Input: part model. Units: mm. Frame: model coordinates. Round coordinates to 2 decimals unless told otherwise and drop trailing zeros. Loops run counter-clockwise (first coordinate to the right, second up) from the corner with the lowest first, then second, coordinate; pieces in that order, holes last.
1) Section B-B, the plane y = 0.2. State how many separate pieces and enclosed holes the cut face has, and give its area (3 significant figures).
2) Section A-A, the plane x = 11.5. Return loops of the section in (y, z) (3 decimals), and give its area (3 significant figures).
3) First-contact query: pin 1 (0.6 mm diameter, centred on x = -26.5, y = 1, fed in from +Z); pin 2 (0.6 mm diameter, centred on x = -28, y = 0.5, fed in from -Z). Flat tips, straight axial feed; report the tip coordinate or a pass-through.
4) Ray query, line 1 along Z through (x, y) = (-25, 0.1); line 2 along X through (y, z) = (0, 7); line 3 along Z through (x, y) = (2.5, 1). Return the intervals inside material, ascending.
from build123d import *

# Parameters (mm, degrees)
SKETCH1_R           = 7.6
BOSS_EXTRUDE1_DEPTH = 1.8
FILLET1_R           = 3
FILLET2_R           = 1.4
SCALE1_SCALE        = 1.15


with BuildPart() as part:
    # Sketch1 → Boss-Extrude1 (new body)
    with BuildSketch(Plane(origin=(0, 0, 0), x_dir=(1, 0, 0), z_dir=(0, 1, 0))):
        Polygon((20.3, 35.160631394), (-20.3, 35.160631394), (-40.6, 0), (-20.3, -35.160631394), (20.3, -35.160631394), (40.6, 0), align=None)
        Polygon((-16.584596387, -31.040676977), (-16.771232891, -33.649562724), (-19.310104532, -34.278250893), (-20.692576995, -32.057915803), (-19.008120326, -30.056985082), align=None, mode=Mode.SUBTRACT)
        Polygon((-35.174313007, -1.157656706), (-37.526992591, -2.300467626), (-39.340888337, -0.416084372), (-38.109257976, 1.891339446), (-35.534172805, 1.433022539), align=None, mode=Mode.SUBTRACT)
        Polygon((18.589716619, -29.883020272), (20.7557597, -31.349095098), (20.030783805, -33.862166521), (17.41668098, -33.94925525), (16.52605248, -31.490007621), align=None, mode=Mode.SUBTRACT)
        with BuildLine():
            Line((-32.142053523, 3.218057696), (-18.857946477, 26.226806032))
            Line((-18.857946477, 26.226806032), (-10.521325069, 11.78735419))
            ThreePointArc((-10.521325069, 11.78735419), (-13.68320138, 7.9), (-15.468810706, 3.218057696))
            Line((-15.468810706, 3.218057696), (-32.142053523, 3.218057696))
        make_face(mode=Mode.SUBTRACT)
        with BuildLine():
            Line((-18.857946477, -26.226806032), (-32.142053523, -3.218057696))
            Line((-32.142053523, -3.218057696), (-15.468810706, -3.218057696))
            ThreePointArc((-15.468810706, -3.218057696), (-13.68320138, -7.9), (-10.521325069, -11.78735419))
            Line((-10.521325069, -11.78735419), (-18.857946477, -26.226806032))
        make_face(mode=Mode.SUBTRACT)
        with BuildLine():
            Line((13.284107046, -29.444863729), (-13.284107046, -29.444863729))
            Line((-13.284107046, -29.444863729), (-4.947485637, -15.005411886))
            ThreePointArc((-4.947485637, -15.005411886), (0, -15.8), (4.947485637, -15.005411886))
            Line((4.947485637, -15.005411886), (13.284107046, -29.444863729))
        make_face(mode=Mode.SUBTRACT)
        with BuildLine():
            Line((32.142053523, -3.218057696), (18.857946477, -26.226806032))
            Line((18.857946477, -26.226806032), (10.521325069, -11.78735419))
            ThreePointArc((10.521325069, -11.78735419), (13.68320138, -7.9), (15.468810706, -3.218057696))
            Line((15.468810706, -3.218057696), (32.142053523, -3.218057696))
        make_face(mode=Mode.SUBTRACT)
        with BuildLine():
            Line((18.857946477, 26.226806032), (32.142053523, 3.218057696))
            Line((32.142053523, 3.218057696), (15.468810706, 3.218057696))
            ThreePointArc((15.468810706, 3.218057696), (13.68320138, 7.9), (10.521325069, 11.78735419))
            Line((10.521325069, 11.78735419), (18.857946477, 26.226806032))
        make_face(mode=Mode.SUBTRACT)
        with BuildLine():
            Line((-13.284107046, 29.444863729), (13.284107046, 29.444863729))
            Line((13.284107046, 29.444863729), (4.947485637, 15.005411886))
            ThreePointArc((4.947485637, 15.005411886), (0, 15.8), (-4.947485637, 15.005411886))
            Line((-4.947485637, 15.005411886), (-13.284107046, 29.444863729))
        make_face(mode=Mode.SUBTRACT)
        Polygon((-18.589716619, 29.883020272), (-20.7557597, 31.349095098), (-20.030783805, 33.862166521), (-17.41668098, 33.94925525), (-16.52605248, 31.490007621), align=None, mode=Mode.SUBTRACT)
        Polygon((35.174313007, 1.157656706), (37.526992591, 2.300467626), (39.340888337, 0.416084372), (38.109257976, -1.891339446), (35.534172805, -1.433022539), align=None, mode=Mode.SUBTRACT)
        Polygon((16.584596387, 31.040676977), (16.771232891, 33.649562724), (19.310104532, 34.278250893), (20.692576995, 32.057915803), (19.008120326, 30.056985082), align=None, mode=Mode.SUBTRACT)
        with Locations(Location((0.052857117, 0, 0), (0, 0, 270))):
            Circle(SKETCH1_R, mode=Mode.SUBTRACT)
    extrude(amount=BOSS_EXTRUDE1_DEPTH)

    # Fillet1
    # the kernel refuses this fillet: 3 mm, written as the material it takes off along each edge
    with BuildSketch(Plane(origin=(40.6, -4.330127019, 0), x_dir=(-0.4999999999998131, 0, -0.8660254037845465), z_dir=(0, 1, 0))) as fillet1_piece_1:
        with BuildLine():
            CenterArc((FILLET1_R * 0.577350269186, FILLET1_R), FILLET1_R, 210, 60)
            Line((-FILLET1_R * 0.288675134596, FILLET1_R * 0.499999999995), (0, 0))
            Line((0, 0), (FILLET1_R * 0.577350269186, 0))
        make_face()
    extrude(amount=10.460254038, mode=Mode.SUBTRACT)
    with BuildSketch(Plane(origin=(20.3, -4.330127019, 35.160631394), x_dir=(-1.0, 0, -2.4203690345734148e-12), z_dir=(0, 1, 0)), Plane(origin=(-20.3, -4.330127019, 35.160631394), x_dir=(-0.5000000000021431, 0, -0.8660254037832013), z_dir=(0, 1, 0)), Plane(origin=(-40.6, -4.330127019, 0), x_dir=(0.49999999999780936, 0, -0.8660254037857034), z_dir=(0, 1, 0)), Plane(origin=(-20.3, -4.330127019, -35.160631394), x_dir=(1, 0, 0), z_dir=(0, 1, 0)), Plane(origin=(20.3, -4.330127019, -35.160631394), x_dir=(0.49999999999981115, 0, 0.8660254037845477), z_dir=(0, 1, 0))) as fillet1_piece_2:
        with BuildLine():
            CenterArc((FILLET1_R * 0.577350269195, -FILLET1_R), FILLET1_R, 90, 60)
            Line((-FILLET1_R * 0.288675134594, -FILLET1_R * 0.500000000007), (0, 0))
            Line((0, 0), (FILLET1_R * 0.577350269195, 0))
        make_face()
    extrude(amount=10.460254038, mode=Mode.SUBTRACT)

    # Fillet2
    fillet2_edges = [part.edges().sort_by_distance(p)[0] for p in [
        (-32.142053523, 0.9, -3.218057696),
        (-15.468810706, 0.9, -3.218057696),
        (-10.521325069, 0.9, -11.78735419),
        (-18.857946477, 0.9, -26.226806032),
        (-18.857946477, 0.9, 26.226806032),
        (-10.521325069, 0.9, 11.78735419),
        (-15.468810706, 0.9, 3.218057696),
        (-32.142053523, 0.9, 3.218057696),
        (13.284107046, 0.9, 29.444863729),
        (4.947485637, 0.9, 15.005411886),
        (-4.947485637, 0.9, 15.005411886),
        (-13.284107046, 0.9, 29.444863729),
        (32.142053523, 0.9, 3.218057696),
        (15.468810706, 0.9, 3.218057696),
        (10.521325069, 0.9, 11.78735419),
        (18.857946477, 0.9, 26.226806032),
        (18.857946477, 0.9, -26.226806032),
        (10.521325069, 0.9, -11.78735419),
        (15.468810706, 0.9, -3.218057696),
        (32.142053523, 0.9, -3.218057696),
        (-13.284107046, 0.9, -29.444863729),
        (-4.947485637, 0.9, -15.005411886),
        (4.947485637, 0.9, -15.005411886),
        (13.284107046, 0.9, -29.444863729),
    ]]
    fillet(fillet2_edges, radius=FILLET2_R)


with BuildPart() as part_1:
    # Scale1: scaled about (-0.00383883, 0.9, 0)
    add(part.part.scale(SCALE1_SCALE).moved(Location((0.000575824, -0.135, 0))))


solid = part_1.part
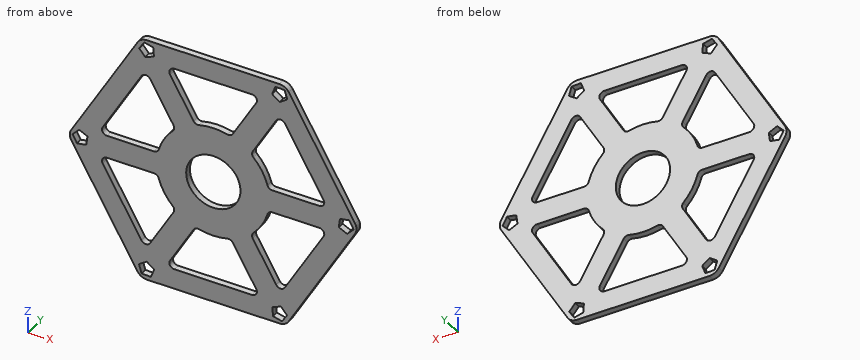
Final values:
1. separate pieces: 1
1. enclosed holes: 13
1. area: 3,300 mm2
2. outline: (-0.135, -40.435) - (1.935, -40.435) - (1.935, -33.862) - (-0.135, -33.862) - close; (-0.135, -27.319) - (1.935, -27.319) - (1.935, 27.319) - (-0.135, 27.319) - close; (-0.135, 33.862) - (1.935, 33.862) - (1.935, 40.435) - (-0.135, 40.435) - close
2. area: 140 mm2
3. pin 1: stops at z = 35.49
3. pin 2: stops at z = -32.89
4. line 1: z = -37.57 to -24.42, -3.7 to 3.7, 24.42 to 37.57
4. line 2: x = -42.65 to -35.06, -16.77 to -5.17, 5.29 to 16.77, 35.06 to 42.65
4. line 3: z = -40.43 to -33.86, -18 to -8.39, 8.39 to 18, 33.86 to 40.43
